```python
from build123d import *

# Parameters (mm, degrees)
IZIM1_R                          = 2.5
Y_KSEKLIK_EKSTR_ZYON1_DEPTH      = 2
IZIM2_W                          = 25
IZIM2_H                          = 31
Y_KSEKLIK_EKSTR_ZYON2_DEPTH      = 2
IZIM3_W                          = 0.888238836
IZIM3_H                          = 3.17016103
KES_EKSTR_ZYON1_DEPTH            = 2
IZIM6_W                          = 3
IZIM6_H                          = 31
Y_KSEKLIK_EKSTR_ZYON3_DEPTH      = 10
IZIM7_R                          = 1.6
KES_EKSTR_ZYON2_DEPTH            = 141
IZIM8_W                          = 4.55247788
IZIM8_H                          = 5.743045402
Y_KSEKLIK_EKSTR_ZYON4_DEPTH      = 2
Y_KSEKLIK_EKSTR_ZYON5_DEPTH      = 31
Y_KSEKLIK_EKSTR_ZYON6_REACH      = 85.274
Y_KSEKLIK_EKSTR_ZYON6_END_RADIUS = 43.5625
RADYUS1_R                        = 3
RADYUS2_R                        = 2
IZIM11_W                         = 25
IZIM11_H                         = 20
KES_EKSTR_ZYON3_DEPTH            = 10
Y_KSEKLIK_EKSTR_ZYON7_DEPTH      = 2


with BuildPart() as part:
    # Çizim1 → Yükseklik-Ekstrüzyon1 (new body)
    with BuildSketch(Plane.XY):
        with BuildLine():
            Line((-11.5, 17.5), (11.5, 17.5))
            ThreePointArc((11.5, 17.5), (12.914213562, 16.914213562), (13.5, 15.5))
            Line((13.5, 15.5), (13.5, -15.5))
            ThreePointArc((13.5, -15.5), (12.914213562, -16.914213562), (11.5, -17.5))
            Line((11.5, -17.5), (-11.5, -17.5))
            ThreePointArc((-11.5, -17.5), (-12.914213562, -16.914213562), (-13.5, -15.5))
            Line((-13.5, -15.5), (-13.5, 15.5))
            ThreePointArc((-13.5, 15.5), (-12.914213562, 16.914213562), (-11.5, 17.5))
        make_face()
        with Locations((-10, 14)):
            Circle(IZIM1_R, mode=Mode.SUBTRACT)
        with Locations((-10, -14)):
            Circle(IZIM1_R, mode=Mode.SUBTRACT)
        with Locations((10, 14)):
            Circle(IZIM1_R, mode=Mode.SUBTRACT)
        with Locations((10, -14)):
            Circle(IZIM1_R, mode=Mode.SUBTRACT)
    y_kseklik_ekstr_zyon1 = extrude(amount=Y_KSEKLIK_EKSTR_ZYON1_DEPTH)

    # Çizim2 → Yükseklik-Ekstrüzyon2 (add)
    with BuildSketch(Plane(origin=(0, 0, 0), x_dir=(-1, 0, 0), z_dir=(0, 0, -1))):
        with Locations((26, 0)):
            Rectangle(IZIM2_W, IZIM2_H)
    extrude(amount=-Y_KSEKLIK_EKSTR_ZYON2_DEPTH)

    # Çizim3 → Kes-Ekstrüzyon1 (cut)
    with BuildSketch(Plane(origin=(0, 0, 0), x_dir=(-1, 0, 0), z_dir=(0, 0, -1))):
        with Locations((26.444119418, 13.914919485)):
            Rectangle(IZIM3_W, IZIM3_H)
    extrude(amount=-KES_EKSTR_ZYON1_DEPTH, mode=Mode.SUBTRACT)

    # Aynalama4: Yükseklik-Ekstrüzyon1 across plane
    add(y_kseklik_ekstr_zyon1.mirror(Plane(origin=(-26, 15.5, 2), x_dir=(0, 0, 1), z_dir=(1, 0, 0))))

    # Çizim6 → Yükseklik-Ekstrüzyon3 (add)
    with BuildSketch(Plane(origin=(0, 0, 0), x_dir=(-1, 0, 0), z_dir=(0, 0, -1))):
        with Locations((-15, 0)):
            Rectangle(IZIM6_W, IZIM6_H)
        with Locations((67, 0)):
            Rectangle(IZIM6_W, IZIM6_H)
    extrude(amount=-Y_KSEKLIK_EKSTR_ZYON3_DEPTH)

    # Çizim7 → Kes-Ekstrüzyon2 (cut)
    with BuildSketch(Plane(origin=(16.5, 0, 0), x_dir=(0, 0, -1), z_dir=(1, 0, 0))):
        with Locations((-6.681859939, 11.575153699)):
            Circle(IZIM7_R)
        with Locations((-6.681859939, 0)):
            Circle(IZIM7_R)
        with Locations((-6.681859939, -12.069818387)):
            Circle(IZIM7_R)
    extrude(amount=-KES_EKSTR_ZYON2_DEPTH, mode=Mode.SUBTRACT)

    # Çizim8 → Yükseklik-Ekstrüzyon4 (add)
    with BuildSketch(Plane(origin=(0, 0, 0), x_dir=(-1, 0, 0), z_dir=(0, 0, -1))):
        with Locations((26.803888867, 12.628477299)):
            Rectangle(IZIM8_W, IZIM8_H)
    extrude(amount=-Y_KSEKLIK_EKSTR_ZYON4_DEPTH)

    # Çizim9 → Yükseklik-Ekstrüzyon5 (add)
    with BuildSketch(Plane.XZ.offset(15.5)):
        with BuildLine():
            Line((-68.5, 10), (-65.5, 10))
            ThreePointArc((-65.5, 10), (-26, 42), (13.5, 10))
            Line((13.5, 10), (16.5, 10))
            ThreePointArc((16.5, 10), (-26, 44), (-68.5, 10))
        make_face()
    extrude(amount=-Y_KSEKLIK_EKSTR_ZYON5_DEPTH)

    # Yükseklik-Ekstrüzyon6: up to this cylinder (the profile starts inside it)
    y_kseklik_ekstr_zyon6_end = Plane(origin=(-26, 18.142911, 0.4375), z_dir=(0, -1, 0)) * Cylinder(Y_KSEKLIK_EKSTR_ZYON6_END_RADIUS, 258.673, mode=Mode.PRIVATE)
    # Çizim10 → Yükseklik-Ekstrüzyon6 (add, up to the surface)
    with BuildSketch(Plane(origin=(0, 0, 0), x_dir=(-1, 0, 0), z_dir=(0, 0, -1)), mode=Mode.PRIVATE) as y_kseklik_ekstr_zyon6_sk1:
        with BuildLine():
            Line((68.5, 19.845287322), (68.5, 15.5))
            Line((68.5, 15.5), (65.5, 15.5))
            ThreePointArc((65.5, 15.5), (64.914213562, 16.914213562), (63.5, 17.5))
            Line((63.5, 17.5), (40.5, 17.5))
            ThreePointArc((40.5, 17.5), (39.085786438, 16.914213562), (38.5, 15.5))
            Line((38.5, 15.5), (13.5, 15.5))
            ThreePointArc((13.5, 15.5), (12.914213562, 16.914213562), (11.5, 17.5))
            Line((11.5, 17.5), (-11.5, 17.5))
            ThreePointArc((-11.5, 17.5), (-12.914213562, 16.914213562), (-13.5, 15.5))
            Line((-13.5, 15.5), (-16.5, 15.5))
            Line((-16.5, 15.5), (-16.5, 19.845287322))
            Line((-16.5, 19.845287322), (68.5, 19.845287322))
        make_face()
    y_kseklik_ekstr_zyon6_tool1 = extrude(y_kseklik_ekstr_zyon6_sk1.sketch, amount=-Y_KSEKLIK_EKSTR_ZYON6_REACH, mode=Mode.PRIVATE) & y_kseklik_ekstr_zyon6_end
    add(y_kseklik_ekstr_zyon6_tool1.solids().sort_by_distance((-26, 18.142911, 0))[0])

    # Radyus1
    # the kernel refuses this fillet: 3 mm, written as the material it takes off along each edge
    with BuildSketch(Plane(origin=(-68.5, 19.845287322, -7.5), x_dir=(1, 0, 0), z_dir=(0, 0, 1)), Plane(origin=(16.5, 19.845287322, -7.5), x_dir=(0, -1, 0), z_dir=(0, 0, 1))) as radyus1_piece_1:
        with BuildLine():
            CenterArc((RADYUS1_R, -RADYUS1_R), RADYUS1_R, 90, 90)
            Line((0, -RADYUS1_R), (0, 0))
            Line((0, 0), (RADYUS1_R, 0))
        make_face()
    extrude(amount=25, mode=Mode.SUBTRACT)
    with BuildSketch(Plane(origin=(-26, 19.845287322, 0.4375), x_dir=(0.9988024950915276, 0, 0.04892418419288032), z_dir=(0.04892418419288032, 0, -0.9988024950915276))) as radyus1_piece_2:
        with BuildLine():
            CenterArc((43.5625 - RADYUS1_R, RADYUS1_R), RADYUS1_R, 270, 90)
            Line((43.5625 - RADYUS1_R, 0), (43.5625, 0))
            Line((43.5625, 0), (43.5625, RADYUS1_R))
        make_face()
    revolve(axis=Axis((-26, 19.845287322, 0.4375), (0, -1, 0)), revolution_arc=174.39146253, mode=Mode.SUBTRACT)

    # Radyus2
    radyus2_edges = [part.edges().sort_by_distance(p)[0] for p in [
        (-68.5, 0.672643661, 0),
        (-26, 19.845287322, 0),
        (16.5, 0.672643661, 0),
        (-67.621320344, 18.966607666, 0),
        (15.621320344, 18.966607666, 0),
    ]]
    fillet(radyus2_edges, radius=RADYUS2_R)

    # Çizim11 → Kes-Ekstrüzyon3 (cut)
    with BuildSketch(Plane(origin=(0, 0, 0), x_dir=(-1, 0, 0), z_dir=(0, 0, -1))):
        with Locations((51.5, 1)):
            Rectangle(IZIM11_W, IZIM11_H)
        with Locations((0.5, 1)):
            Rectangle(IZIM11_W, IZIM11_H)
    extrude(amount=-KES_EKSTR_ZYON3_DEPTH, mode=Mode.SUBTRACT)

    # Çizim12 → Yükseklik-Ekstrüzyon7 (add)
    with BuildSketch(Plane(origin=(0, 0, 0), x_dir=(-1, 0, 0), z_dir=(0, 0, -1))):
        with BuildLine():
            Line((11.5, -17.5), (40.5, -17.5))
            ThreePointArc((40.5, -17.5), (39.085786438, -16.914213562), (38.5, -15.5))
            Line((38.5, -15.5), (13.5, -15.5))
            ThreePointArc((13.5, -15.5), (12.914213562, -16.914213562), (11.5, -17.5))
        make_face()
    extrude(amount=-Y_KSEKLIK_EKSTR_ZYON7_DEPTH)


solid = part.part
```
Input: part model. Units: mm. Frame: model coordinates. A direction names the side the tool comes from. Round coordinates to 2 decimals unless told otherwise and drop trailing zeros. Loops run counter-clockwise (first coordinate to the right, second up) from the corner with the lowest first, then second, coordinate; pieces in that order, holes last. Notation, with made-up numbers: (23.5, 54) - (58.5, 54) arc R23 ccw to (58.5, 89) - close; hole circle Ø11 at (14.25, 7). An arc over 180 degrees is marked (long way). One line per item, written item: value. Start each with the question number.
(1) Section D-D, the plane z = 25. Count the separate pieces of the cut face and the enclosed holes in it, plus the area to 3 significant figures.
(2) Section C-C, the plane y = 0. Return loops of the section in (x, z) (1 decimal).
(3) Ray query, line 1 (Y direction, x = -42, z = 1.3); line 2 (X direction, y = 8.5, z = 5); line 3 (Y direction, x = -17, z = 14.5). Return the intervals inside material, ascending. Write a range as [from, to].
(4) Section A-A, the plane y = 14. Return loops of the section in (x, z) (1 decimal).
(5) Contact query for flat-ended pins moving along their axis: P1, Ø8, axis at x = -9, z = 7.5, coming from the -Y side; P2, Ø12, axis at x = -54, z = 28.5, coming from the -Y side; P3, Ø4, axis at x = -10, y = -14, coming from the -Z side. Output: stop coordinate, or through.
(6) Access query for faces 1 (the flat face through (12, 1, 1)), 2 (the flat face through (-25, -17.5, 1)). Directions: +Z, -Z, +X, -X, +Y, -Y. A direction counts if a zero-diameter tool reaches every point of the face in a straight line with its end or side. Return the directions, or none.
(7) Draft query along Y for faces 3 (the cylindrical face through (-64.385, 14.751, 0.986)), 4 (the flat face through (-26, 15.5, 22)), 5 (the cylindrical face through (-66.98, 12.66, 7.86)), 6 (the flat face through (13.5, 0, 4)). Return one class per face: +Y half, -Y half, draft (parallel to the pull), parting line (faces both ways), or undercut.
(8) Section B-B, the plane y = -6.5. Return loops of the section in (x, z) (1 decimal).
Results below:
1. separate pieces: 3
1. enclosed holes: 0
1. area: 405 mm^2
2. outline: (-68.5, 2) arc R2 ccw to (-66.5, 0) - (-64, 0) - (-64, 2) - (-65.5, 2) - (-65.5, 5.1) - (-68.5, 5.1) - close; (-68.5, 8.3) - (-65.5, 8.3) - (-65.5, 10) arc R40.4 cw to (13.5, 10) - (13.5, 8.3) - (16.5, 8.3) - (16.5, 10) arc R43.6 ccw to (-68.5, 10) - close; (-39, 0) - (-13, 0) - (-13, 2) - (-39, 2) - close; (12, 0) - (14.5, 0) arc R2 ccw to (16.5, 2) - (16.5, 5.1) - (13.5, 5.1) - (13.5, 2) - (12, 2) - close
3. line 1: [-17.5, -16.5], [-11.5, -9], [11, 11.5], [16.5, 19.72]
3. line 2: [-68.5, -65.5], [13.5, 16.5]
3. line 3: [15.5, 19.85]
4. outline: (-68.5, 2) arc R2 ccw to (-66.5, 0) - (-64.5, 0) - (-64.5, 2) - (-65.5, 2) - (-65.5, 10) arc R40.4 cw to (13.5, 10) - (13.5, 2) - (12.5, 2) - (12.5, 0) - (14.5, 0) arc R2 ccw to (16.5, 2) - (16.5, 10) arc R43.6 ccw to (-68.5, 10) - close; (-59.5, 0) - (-44.5, 0) - (-44.5, 2) - (-59.5, 2) - close; (-39.5, 0) - (-12.5, 0) - (-12.5, 2) - (-39.5, 2) - close; (-7.5, 0) - (7.5, 0) - (7.5, 2) - (-7.5, 2) - close
5. P1: y = 16.82
5. P2: y = -15.5
5. P3: z = 37.77
6. face 1: -Z
6. face 2: +Z, -Z, +X, -X, -Y
7. face 3: undercut
7. face 4: -Y half
7. face 5: undercut
7. face 6: draft
8. outline: (-68.5, 2) arc R2 ccw to (-66.5, 0) - (-64, 0) - (-64, 2) - (-65.5, 2) - (-65.5, 10) arc R40.4 cw to (13.5, 10) - (13.5, 2) - (12, 2) - (12, 0) - (14.5, 0) arc R2 ccw to (16.5, 2) - (16.5, 10) arc R43.6 ccw to (-68.5, 10) - close; (-39, 0) - (-13, 0) - (-13, 2) - (-39, 2) - close
